from build123d import *

# Parameters (mm, degrees)
CROQUIS1_R              = 39.5
CROQUIS1_R_2            = 12.5
CROQUIS1_R_3            = 2
SALIENTE_EXTRUIR1_DEPTH = 28
CROQUIS3_R              = 15
CORTAR_EXTRUIR1_DEPTH   = 12
CROQUIS5_R              = 16.857920318
SALIENTE_EXTRUIR2_DEPTH = 10
CROQUIS4_R              = 1.75
CORTAR_EXTRUIR2_DEPTH   = 10


with BuildPart() as part:
    # Croquis1 → Saliente-Extruir1 (new body)
    with BuildSketch(Plane.XY):
        Circle(CROQUIS1_R)
        Circle(CROQUIS1_R_2, mode=Mode.SUBTRACT)
        with Locations((0, 30)):
            Circle(CROQUIS1_R_3, mode=Mode.SUBTRACT)
        with Locations((30, 0)):
            Circle(CROQUIS1_R_3, mode=Mode.SUBTRACT)
        with Locations((0, -30)):
            Circle(CROQUIS1_R_3, mode=Mode.SUBTRACT)
        with Locations((-30, 0)):
            Circle(CROQUIS1_R_3, mode=Mode.SUBTRACT)
    extrude(amount=SALIENTE_EXTRUIR1_DEPTH)

    # Croquis3 → Cortar-Extruir1 (cut)
    with BuildSketch(Plane.XY.offset(28)):
        Circle(CROQUIS3_R)
        Polygon((17.67766953, 13.435028843), (25.455844123, 21.213203436), (21.213203436, 25.455844123), (13.435028843, 17.67766953), align=None)
        Polygon((13.435028843, -17.67766953), (21.213203436, -25.455844123), (25.455844123, -21.213203436), (17.67766953, -13.435028843), align=None)
        Polygon((-17.67766953, -13.435028843), (-25.455844123, -21.213203436), (-21.213203436, -25.455844123), (-13.435028843, -17.67766953), align=None)
        Polygon((-13.435028843, 17.67766953), (-21.213203436, 25.455844123), (-25.455844123, 21.213203436), (-17.67766953, 13.435028843), align=None)
    extrude(amount=-CORTAR_EXTRUIR1_DEPTH, mode=Mode.SUBTRACT)

    # Croquis5 → Saliente-Extruir2 (add)
    with BuildSketch(Plane(origin=(0, 0, 0), x_dir=(-1, 0, 0), z_dir=(0, 0, -1))):
        Circle(CROQUIS5_R)
    extrude(amount=-SALIENTE_EXTRUIR2_DEPTH)

    # Croquis4 → Cortar-Extruir2 (cut)
    with BuildSketch(Plane(origin=(0, 0, 0), x_dir=(-1, 0, 0), z_dir=(0, 0, -1))):
        with Locations((-12.727922061, -6.363961031)):
            Circle(CROQUIS4_R)
        with Locations((-6.363961031, -12.727922061)):
            Circle(CROQUIS4_R)
        with Locations((21.920310217, 28.284271247)):
            Circle(CROQUIS4_R)
        with Locations((28.284271247, 21.920310217)):
            Circle(CROQUIS4_R)
        Polygon((30, -3.5), (33.031088913, -1.75), (33.031088913, 1.75), (30, 3.5), (26.968911087, 1.75), (26.968911087, -1.75), align=None)
        Polygon((3.5, 30), (1.75, 33.031088913), (-1.75, 33.031088913), (-3.5, 30), (-1.75, 26.968911087), (1.75, 26.968911087), align=None)
        Polygon((-3.5, -30), (-1.75, -33.031088913), (1.75, -33.031088913), (3.5, -30), (1.75, -26.968911087), (-1.75, -26.968911087), align=None)
        Polygon((-30, 3.5), (-33.031088913, 1.75), (-33.031088913, -1.75), (-30, -3.5), (-26.968911087, -1.75), (-26.968911087, 1.75), align=None)
        Polygon((0.353553391, -13.788582233), (29.344931419, 15.202795796), (15.202795796, 29.344931419), (-13.788582233, 0.353553391), align=None)
    extrude(amount=-CORTAR_EXTRUIR2_DEPTH, mode=Mode.SUBTRACT)


solid = part.part
The listing builds one solid part. Answer for the finished solid, in the listing's coordinates (mm). A direction names the side the tool comes from. Round coordinates to 2 decimals unless told otherwise and drop trailing zeros. Order: outer loops, then holes, each group sorted by start corner. A loop starts at its lowest first (then second) coordinate and runs counter-clockwise, first axis right, second up. Notation, with made-up numbers: M 37,43.5 L 56,43.5 A22 cw 56,75.5 Z; hole C -12.75,6.25 d11. An arc over 180 degrees is marked long. Answer in a Markdown table with one row per item. Add a question column.
1) Flat-ended cylindrical pins translate along their axes: pin 1 Ø2 at (x, y) = (12.73, -6.36) entering from -Z; pin 2 Ø3 at (x, z) = (-0.5, 3) entering from +Y; pin 3 Ø5.5 at (x, y) = (-8, -5.5) entering from +Z. Find the tip coordinate at first contact, or state that the pin passes through.
2) Consider line 1 along X through (y, z) = (-16, 17); line 2 along Y through (x, z) = (13, 8.5); line 3 along Y through (x, z) = (9.5, 7). Determine where each line is inside the solid, lowest interval first. Write a range as from..to.
3) The part is cut by section C-C on y = -24. Determine the outline of the cut face in (x, z).
4) The part is cut by section A-A on z = 22.75. Count the separate pieces of the cut face and the enclosed holes in it, plus the area to 3 significant figures.
5) The part is cut by section B-B on x = -8. Determine the outline of the cut face in (y, z), plus the area to 3 significant figures.
6) Which of the six approach directions +Z, -Z, +X, -X, +Y, -Y give full straight-line access (tool end or side, diameter ignored) to faces 1 (the face through (-14.985, 0.66, 22.084)), 2 (the face through (0, -32, 19)), 3 (the face through (-22, 28, 10))?
Findings below:
| question | item | result |
|---|---|---|
| 1 | pin 1 | stops at z = 10 |
| 1 | pin 2 | stops at y = 39.5 |
| 1 | pin 3 | stops at z = 10 |
| 2 | line 1 | x = -36.11..-20.24, -15.11..15.11, 20.24..36.11 |
| 2 | line 2 | y = -37.3..-8.09, -4.64..-0.44, 1.14..37.3 |
| 2 | line 3 | y = -38.34..-3.94, 4.64..38.34 |
| 3 | outline | M -31.37,0 L 31.37,0 L 31.37,28 L 22.67,28 L 22.67,16 L 19.76,16 L 19.76,28 L -19.76,28 L -19.76,16 L -22.67,16 L -22.67,28 L -31.37,28 Z |
| 4 | separate pieces | 1 |
| 4 | enclosed holes | 9 |
| 4 | area | 3,880 mm² |
| 5 | outline | M -38.68,0 L -6.14,0 L -6.14,10 L -9.6,10 L -9.6,16 L -12.69,16 L -12.69,28 L -38.68,28 Z; M 9.6,10 L 22.14,10 L 22.14,0 L 38.68,0 L 38.68,28 L 12.69,28 L 12.69,16 L 9.6,16 Z |
| 5 | area | 1,460 mm² |
| 6 | face 1 | +Z |
| 6 | face 2 | +Z, -Z |
| 6 | face 3 | -Z |
